Geometry: final body of the model. Coordinates: model frame, mm. A direction names the side the tool comes from. Coordinates: 2 decimals unless noted, no trailing zeros. Order: outer loops, then holes, each group sorted by start corner. A loop starts at its lowest first (then second) coordinate and runs counter-clockwise, first axis right, second up. Notation, with made-up numbers: (-25.5, 57) -> (-21.5, 57) arc R22 ccw to (-21.5, 67) -> close; hole circle Ø6 at (-4.5, 21.25). An arc over 180 degrees is marked (long way). Use one line per item in the form item = value.
```python
from build123d import *

# Parameters (mm, degrees)
SKETCH1_W           = 149
SKETCH1_H           = 51
SKETCH1_W_2         = 137
SKETCH1_H_2         = 39
EXTRUDE_THIN1_DEPTH = 25.5
SKETCH2_W           = 146
SKETCH2_H           = 48
CUT_EXTRUDE1_DEPTH  = 3
CUT_EXTRUDE2_DEPTH  = 8
CUT_EXTRUDE3_DEPTH  = 8
FILLET1_R           = 2
FILLET2_R           = 2
CUT_EXTRUDE7_DEPTH  = 14


with BuildPart() as part:
    # Sketch1 → Extrude-Thin1 (new body)
    with BuildSketch(Plane.XY):
        with Locations((74.5, 25.5)):
            Rectangle(SKETCH1_W, SKETCH1_H)
        with Locations((74.5, 25.5)):
            Rectangle(SKETCH1_W_2, SKETCH1_H_2, mode=Mode.SUBTRACT)
    extrude(amount=EXTRUDE_THIN1_DEPTH)

    # Sketch2 → Cut-Extrude1 (cut)
    with BuildSketch(Plane.XY.offset(25.5)):
        with Locations((74.5, 25.5)):
            Rectangle(SKETCH2_W, SKETCH2_H)
    extrude(amount=-CUT_EXTRUDE1_DEPTH, mode=Mode.SUBTRACT)

    # Sketch3 → Cut-Extrude2 (cut)
    with BuildSketch(Plane.XY.offset(22.5)):
        with BuildLine():
            ThreePointArc((4.5, 45), (5.560660172, 45.439339828), (6, 46.5))
            Line((6, 46.5), (4.5, 46.5))
            Line((4.5, 46.5), (4.5, 45))
        make_face()
        with BuildLine():
            Line((4.5, 46.5), (6, 46.5))
            ThreePointArc((6, 46.5), (3.439339828, 47.560660172), (4.5, 45))
            Line((4.5, 45), (4.5, 46.5))
        make_face()
        with BuildLine():
            ThreePointArc((4.5, 45), (5.560660172, 45.439339828), (6, 46.5))
            Line((6, 46.5), (4.5, 46.5))
            Line((4.5, 46.5), (4.5, 45))
        make_face()
        with BuildLine():
            Line((4.5, 46.5), (6, 46.5))
            ThreePointArc((6, 46.5), (3.439339828, 47.560660172), (4.5, 45))
            Line((4.5, 45), (4.5, 46.5))
        make_face()
        with BuildLine():
            ThreePointArc((6, 4.5), (5.560660172, 5.560660172), (4.5, 6))
            Line((4.5, 6), (4.5, 4.5))
            Line((4.5, 4.5), (6, 4.5))
        make_face()
        with BuildLine():
            Line((4.5, 4.5), (4.5, 6))
            ThreePointArc((4.5, 6), (3.439339828, 3.439339828), (6, 4.5))
            Line((6, 4.5), (4.5, 4.5))
        make_face()
        with BuildLine():
            ThreePointArc((6, 4.5), (5.560660172, 5.560660172), (4.5, 6))
            Line((4.5, 6), (4.5, 4.5))
            Line((4.5, 4.5), (6, 4.5))
        make_face()
        with BuildLine():
            Line((4.5, 4.5), (4.5, 6))
            ThreePointArc((4.5, 6), (3.439339828, 3.439339828), (6, 4.5))
            Line((6, 4.5), (4.5, 4.5))
        make_face()
        with BuildLine():
            ThreePointArc((146, 46.5), (144.5, 48), (143, 46.5))
            Line((143, 46.5), (144.5, 46.5))
            Line((144.5, 46.5), (144.5, 45))
            ThreePointArc((144.5, 45), (145.560660172, 45.439339828), (146, 46.5))
        make_face()
        with BuildLine():
            Line((144.5, 46.5), (143, 46.5))
            ThreePointArc((143, 46.5), (143.439339828, 45.439339828), (144.5, 45))
            Line((144.5, 45), (144.5, 46.5))
        make_face()
        with BuildLine():
            ThreePointArc((146, 46.5), (144.5, 48), (143, 46.5))
            Line((143, 46.5), (144.5, 46.5))
            Line((144.5, 46.5), (144.5, 45))
            ThreePointArc((144.5, 45), (145.560660172, 45.439339828), (146, 46.5))
        make_face()
        with BuildLine():
            Line((144.5, 46.5), (143, 46.5))
            ThreePointArc((143, 46.5), (143.439339828, 45.439339828), (144.5, 45))
            Line((144.5, 45), (144.5, 46.5))
        make_face()
        with BuildLine():
            ThreePointArc((146, 4.5), (145.560660172, 5.560660172), (144.5, 6))
            Line((144.5, 6), (144.5, 4.5))
            Line((144.5, 4.5), (143, 4.5))
            ThreePointArc((143, 4.5), (144.5, 3), (146, 4.5))
        make_face()
        with BuildLine():
            Line((144.5, 4.5), (144.5, 6))
            ThreePointArc((144.5, 6), (143.439339828, 5.560660172), (143, 4.5))
            Line((143, 4.5), (144.5, 4.5))
        make_face()
        with BuildLine():
            ThreePointArc((146, 4.5), (145.560660172, 5.560660172), (144.5, 6))
            Line((144.5, 6), (144.5, 4.5))
            Line((144.5, 4.5), (143, 4.5))
            ThreePointArc((143, 4.5), (144.5, 3), (146, 4.5))
        make_face()
        with BuildLine():
            Line((144.5, 4.5), (144.5, 6))
            ThreePointArc((144.5, 6), (143.439339828, 5.560660172), (143, 4.5))
            Line((143, 4.5), (144.5, 4.5))
        make_face()
    extrude(amount=-CUT_EXTRUDE2_DEPTH, mode=Mode.SUBTRACT)

    # Sketch4 → Cut-Extrude3 (cut)
    with BuildSketch(Plane(origin=(0, 0, 0), x_dir=(-1, 0, 0), z_dir=(0, 0, -1))):
        with BuildLine():
            ThreePointArc((-146, 46.5), (-144.939339828, 46.939339828), (-144.5, 48))
            Line((-144.5, 48), (-146, 48))
            Line((-146, 48), (-146, 46.5))
        make_face()
        with BuildLine():
            Line((-146, 48), (-144.5, 48))
            ThreePointArc((-144.5, 48), (-147.060660172, 49.060660172), (-146, 46.5))
            Line((-146, 46.5), (-146, 48))
        make_face()
        with BuildLine():
            ThreePointArc((-146, 4.5), (-147.060660172, 1.939339828), (-144.5, 3))
            Line((-144.5, 3), (-146, 3))
            Line((-146, 3), (-146, 4.5))
        make_face()
        with BuildLine():
            Line((-146, 3), (-144.5, 3))
            ThreePointArc((-144.5, 3), (-144.939339828, 4.060660172), (-146, 4.5))
            Line((-146, 4.5), (-146, 3))
        make_face()
        with BuildLine():
            ThreePointArc((-146, 4.5), (-147.060660172, 1.939339828), (-144.5, 3))
            Line((-144.5, 3), (-146, 3))
            Line((-146, 3), (-146, 4.5))
        make_face()
        with BuildLine():
            Line((-146, 3), (-144.5, 3))
            ThreePointArc((-144.5, 3), (-144.939339828, 4.060660172), (-146, 4.5))
            Line((-146, 4.5), (-146, 3))
        make_face()
        with BuildLine():
            ThreePointArc((-146, 46.5), (-144.939339828, 46.939339828), (-144.5, 48))
            Line((-144.5, 48), (-146, 48))
            Line((-146, 48), (-146, 46.5))
        make_face()
        with BuildLine():
            Line((-146, 48), (-144.5, 48))
            ThreePointArc((-144.5, 48), (-147.060660172, 49.060660172), (-146, 46.5))
            Line((-146, 46.5), (-146, 48))
        make_face()
        with BuildLine():
            ThreePointArc((-4.5, 48), (-4.060660172, 46.939339828), (-3, 46.5))
            Line((-3, 46.5), (-3, 48))
            Line((-3, 48), (-4.5, 48))
        make_face()
        with BuildLine():
            Line((-3, 48), (-3, 46.5))
            ThreePointArc((-3, 46.5), (-1.939339828, 46.939339828), (-1.5, 48))
            ThreePointArc((-1.5, 48), (-3, 49.5), (-4.5, 48))
            Line((-4.5, 48), (-3, 48))
        make_face()
        with BuildLine():
            ThreePointArc((-4.5, 48), (-4.060660172, 46.939339828), (-3, 46.5))
            Line((-3, 46.5), (-3, 48))
            Line((-3, 48), (-4.5, 48))
        make_face()
        with BuildLine():
            Line((-3, 48), (-3, 46.5))
            ThreePointArc((-3, 46.5), (-1.939339828, 46.939339828), (-1.5, 48))
            ThreePointArc((-1.5, 48), (-3, 49.5), (-4.5, 48))
            Line((-4.5, 48), (-3, 48))
        make_face()
        with BuildLine():
            Line((-4.5, 3), (-3, 3))
            Line((-3, 3), (-3, 4.5))
            ThreePointArc((-3, 4.5), (-4.060660172, 4.060660172), (-4.5, 3))
        make_face()
        with BuildLine():
            Line((-3, 4.5), (-3, 3))
            Line((-3, 3), (-4.5, 3))
            ThreePointArc((-4.5, 3), (-3, 1.5), (-1.5, 3))
            ThreePointArc((-1.5, 3), (-1.939339828, 4.060660172), (-3, 4.5))
        make_face()
        with BuildLine():
            Line((-4.5, 3), (-3, 3))
            Line((-3, 3), (-3, 4.5))
            ThreePointArc((-3, 4.5), (-4.060660172, 4.060660172), (-4.5, 3))
        make_face()
        with BuildLine():
            Line((-3, 4.5), (-3, 3))
            Line((-3, 3), (-4.5, 3))
            ThreePointArc((-4.5, 3), (-3, 1.5), (-1.5, 3))
            ThreePointArc((-1.5, 3), (-1.939339828, 4.060660172), (-3, 4.5))
        make_face()
    extrude(amount=-CUT_EXTRUDE3_DEPTH, mode=Mode.SUBTRACT)

    # Fillet1
    fillet1_edges = [part.edges().sort_by_distance(p)[0] for p in [
        (1.5, 49.5, 24),
        (147.5, 49.5, 24),
        (147.5, 1.5, 24),
        (1.5, 1.5, 24),
    ]]
    fillet(fillet1_edges, radius=FILLET1_R)

    # Fillet2
    fillet2_edges = [part.edges().sort_by_distance(p)[0] for p in [
        (143, 45, 11.25),
        (6, 45, 11.25),
        (143, 6, 11.25),
        (6, 6, 11.25),
    ]]
    fillet(fillet2_edges, radius=FILLET2_R)

    # Sketch6 → Cut-Extrude7 (cut)
    with BuildSketch(Plane(origin=(0, 0, 0), x_dir=(-1, 0, 0), z_dir=(0, 0, -1))):
        Polygon((-143, 45), (-146.5, 45), (-146.5, 6), (-143, 6), (-143, 2.5), (-6, 2.5), (-6, 6), (-2.5, 6), (-2.5, 45), (-6, 45), (-6, 48.5), (-143, 48.5), align=None)
    extrude(amount=-CUT_EXTRUDE7_DEPTH, mode=Mode.SUBTRACT)


solid = part.part
```
1) Section B-B, the plane y = 34.5. Output: boundary loops of the cut face in (x, z).
Results found:
outline = (0, 0) -> (2.5, 0) -> (2.5, 14) -> (6, 14) -> (6, 22.5) -> (1.5, 22.5) -> (1.5, 25.5) -> (0, 25.5) -> close; (143, 14) -> (146.5, 14) -> (146.5, 0) -> (149, 0) -> (149, 25.5) -> (147.5, 25.5) -> (147.5, 22.5) -> (143, 22.5) -> close
2) Section A-A, the plane x = 92.5. Output: boundary loops of the cut face in (y, z), and give its area (3 significant figures).
Results found:
outline = (0, 0) -> (2.5, 0) -> (2.5, 14) -> (6, 14) -> (6, 22.5) -> (1.5, 22.5) -> (1.5, 25.5) -> (0, 25.5) -> close; (45, 14) -> (48.5, 14) -> (48.5, 0) -> (51, 0) -> (51, 25.5) -> (49.5, 25.5) -> (49.5, 22.5) -> (45, 22.5) -> close
area = 181 mm2
3) Contact query for flat-ended pins moving along their axis: P1, Ø4, axis at x = 4.5, y = 46.5, coming from the -Z side; P2, Ø0.9, axis at x = 144, y = 46, coming from the +Z side. Output: stop coordinate, or through.
Results found:
P1 = 0
P2 = 14.5
4) Section D-D, the plane z = 2. Output: boundary loops of the cut face in (x, y).
Results found:
outline = (0, 0) -> (149, 0) -> (149, 51) -> (0, 51) -> close; hole circle Ø3 at (3, 3); hole circle Ø3 at (3, 48); hole (2.5, 6) -> (6, 6) -> (6, 2.5) -> (143, 2.5) -> (143, 6) -> (146.5, 6) -> (146.5, 45) -> (143, 45) -> (143, 48.5) -> (6, 48.5) -> (6, 45) -> (2.5, 45) -> close; hole circle Ø3 at (146, 3); hole circle Ø3 at (146, 48)
5) Section C-C, the plane z = 12. Output: boundary loops of the cut face in (x, y).
Results found:
outline = (0, 0) -> (149, 0) -> (149, 51) -> (0, 51) -> close; hole (2.5, 6) -> (6, 6) -> (6, 2.5) -> (143, 2.5) -> (143, 6) -> (146.5, 6) -> (146.5, 45) -> (143, 45) -> (143, 48.5) -> (6, 48.5) -> (6, 45) -> (2.5, 45) -> close
6) Access query for faces 4 (the flat face through (6, 47, 7)), 5 (the flat face through (74, 45, 18)), 6 (the flat face through (74, 50, 25.5)), 7 (the flat face through (4, 5, 14.5)). Directions: +Z, -Z, +X, -X, +Y, -Y. A direction counts if a zero-diameter tool reaches every point of the face in a straight line with its end or side. Return the directions, or none.
Results found:
face_4 = -Z
face_5 = +Z, -Z
face_6 = +Z, +X, -X, +Y, -Y
face_7 = +Z
7) Pull-direction query (X, two-part tool) for faces 1 (the flat face through (6, 4, 7)), 2 (the flat face through (73, 51, 13)), 3 (the flat face through (0, 25, 13)); classes: released by +X, released by -X, zero draft, split by the parting line, or undercut.
Results found:
face_1 = undercut
face_2 = zero draft
face_3 = released by -X
8) Material intervals for probe 1 along Y at (x, z) = (146, 3.5); probe 2 along Y at (x, z) = (4.5, 18); probe 3 along X at (y, z) = (48, 4.5), sorted ascending. Write a range as from..to.
Results found:
probe_1 = 0..1.5, 4.5..6, 45..46.5, 49.5..51
probe_2 = 0..3, 6..45, 48..51
probe_3 = 0..1.5, 4.5..6, 143..144.5, 147.5..149
